Could you check a few things on this drawing? It's one solid part, dimensions in mm from its lowest x, y, z. A direction names the side the tool comes from. Coordinates: 2 decimals unless noted, no trailing zeros. Loops run counter-clockwise (first coordinate to the right, second up) from the corner with the lowest first, then second, coordinate; pieces in that order, holes last. Notation, with made-up numbers: (-14.5, 19) -> (43.5, 19) arc R30 ccw to (43.5, 58) -> close; hole circle Ø10 at (63.25, 12). An arc over 180 degrees is marked (long way). One line per question, with ' | ' between items.
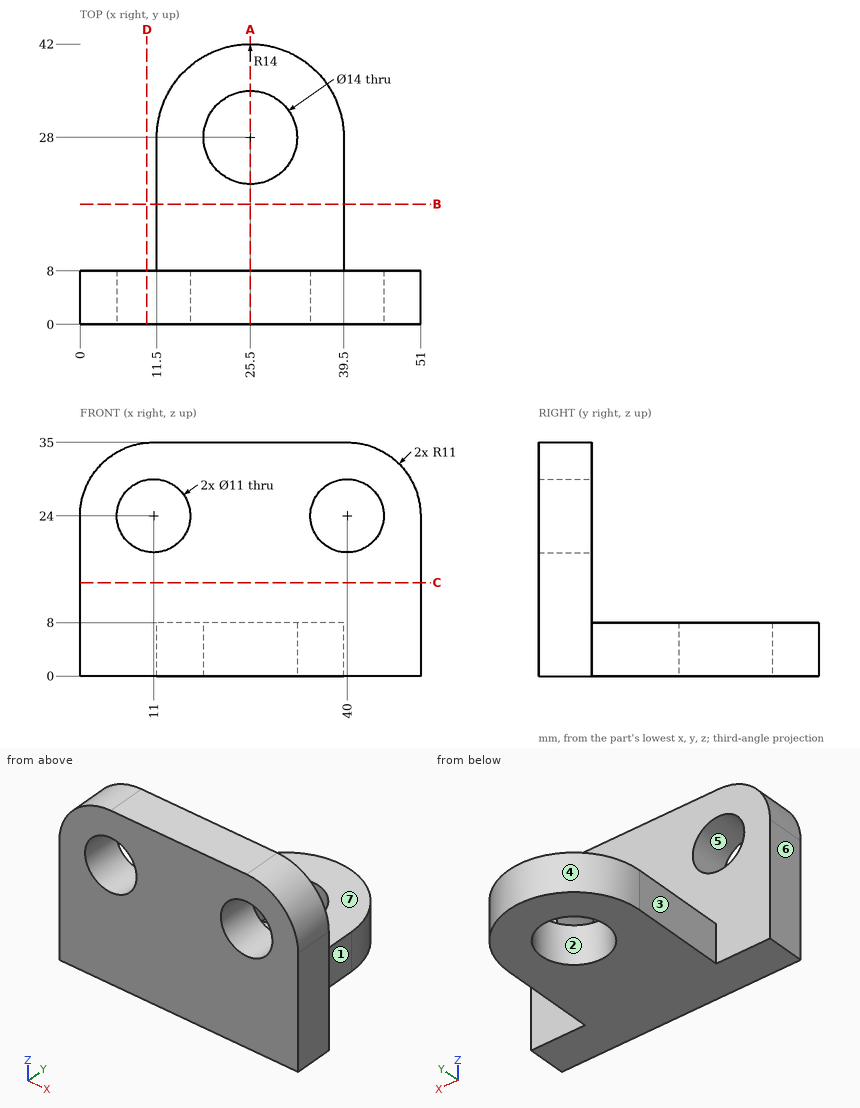
1) I'm going to push flat-ended pins straight in: pin 1 Ø1.5 at (x, y) = (30.5, 27) entering from -Z; pin 2 Ø2 at (x, y) = (39, 24.5) entering from +Z; pin 3 Ø4 at (y, z) = (16, 4.5) entering from +X; pin 4 Ø4 at (y, z) = (23, 3.5) entering from -X. Where does each tip first touch, or does it pass through?
Data:
pin 1: through | pin 2: z = 8 | pin 3: x = 39.5 | pin 4: x = 11.5
2) If we section it at B-B on y = 18: Please give me the cut outline in (x, z), and give its area (3 significant figures).
Data:
outline: (11.5, 0) -> (39.5, 0) -> (39.5, 8) -> (11.5, 8) -> close | area: 224 mm²
3) We'd pull the mould along X, two halves only. Please class the marked faces 4, 5, 6 and 7: pulls with the +X half, pulls with the -X half, needs draft (parallel to the pull), parting line crosses it, or undercut.
Data:
face 4: parting line crosses it | face 5: undercut | face 6: pulls with the -X half | face 7: needs draft
4) If we section it at A-A on x = 25.5: Please give me the cut outline in (y, z), and give its area (3 significant figures).
Data:
outline: (0, 0) -> (21, 0) -> (21, 8) -> (8, 8) -> (8, 35) -> (0, 35) -> close; (35, 0) -> (42, 0) -> (42, 8) -> (35, 8) -> close | area: 440 mm²
5) On a 3-axis mill with a long thin cutter (end or side, diameter ignored), from which of +Z, -Z, +X, -X, +Y, -Y can I reach the whole of each face in a straight line? I mean the marked faces 1, 2 and 3. Say none if no direction works.
Data:
face 1: +Z, -Z, +X, +Y | face 2: +Z, -Z | face 3: +Z, -Z, -X, +Y
6) I need wall thicknesses on line 1 along Y through (x, z) = (25.5, 4); line 2 along X through (y, z) = (15, 5); line 3 along Y through (x, z) = (22, 23.5). Which ranges of each line are inside material? Lowest first, please. Write a range as from..to.
Data:
line 1: 0..21, 35..42 | line 2: 11.5..39.5 | line 3: 0..8
7) If we section it at D-D on x = 10: Please give me the cut outline in (y, z).
Data:
outline: (0, 0) -> (8, 0) -> (8, 18.59) -> (0, 18.59) -> close; (0, 29.41) -> (8, 29.41) -> (8, 34.95) -> (0, 34.95) -> close
8) If we section it at C-C on z = 14: Please give me the cut outline in (x, y).
Data:
outline: (0, 0) -> (51, 0) -> (51, 8) -> (0, 8) -> close
